Check sheet for the modelled part. Datum: model origin and axes. Units: mm. Face numbers are marked on the shaded views. A direction names the side the tool comes from. Coordinates: 2 decimals unless noted, no trailing zeros. Loops run counter-clockwise (first coordinate to the right, second up) from the corner with the lowest first, then second, coordinate; pieces in that order, holes last.
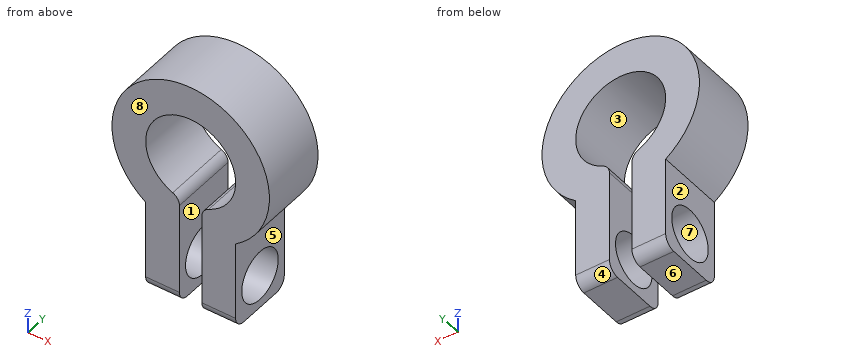
from build123d import *

# Parameters (mm, degrees)
BOSS_EXTRUDE1_DEPTH = 6
SKETCH3_R           = 2.25
CUT_EXTRUDE1_DEPTH  = 10
FILLET1_R           = 1


with BuildPart() as part:
    # Sketch2 → Boss-Extrude1 (new body)
    with BuildSketch(Plane(origin=(0, 0, 0), x_dir=(1, 0, 0), z_dir=(0, 1, 0))):
        with BuildLine():
            Line((-1, 3.872983346), (-1, 13.744562647))
            Line((-1, 13.744562647), (-4, 13.744562647))
            Line((-4, 13.744562647), (-4, 5.744562647))
            ThreePointArc((-4, 5.744562647), (0, -7), (4, 5.744562647))
            Line((4, 5.744562647), (4, 13.744562647))
            Line((4, 13.744562647), (1, 13.744562647))
            Line((1, 13.744562647), (1, 3.872983346))
            ThreePointArc((1, 3.872983346), (0, -4), (-1, 3.872983346))
        make_face()
    extrude(amount=BOSS_EXTRUDE1_DEPTH)

    # Sketch3 → Cut-Extrude1 (cut)
    with BuildSketch(Plane(origin=(4, 0, 0), x_dir=(0, 0, -1), z_dir=(1, 0, 0))):
        with Locations((10.744562647, 3)):
            Circle(SKETCH3_R)
    extrude(amount=-CUT_EXTRUDE1_DEPTH, mode=Mode.SUBTRACT)

    # Fillet1
    fillet1_edges = [part.edges().sort_by_distance(p)[0] for p in [
        (-2.5, 0, -13.744562647),
        (-2.5, 6, -13.744562647),
        (1, 3, -3.872983346),
        (-1, 3, -3.872983346),
        (2.5, 6, -13.744562647),
        (2.5, 0, -13.744562647),
    ]]
    fillet(fillet1_edges, radius=FILLET1_R)


solid = part.part
(1) Draft check along Y on the marked faces 6, 7 and 8. Enter one of: pulls with the +Y half, pulls with the -Y half, needs draft (parallel to the pull), parting line crosses it, or undercut.
(2) Section check D-D, the plane x = -1.25. Enter the section's corners in (y, z), plus the area to 3 significant figures.
(3) Scan lines: line 1 along X through (y, z) = (5.3, -11); line 2 along Z through (x, y) = (-1.75, 1.55); line 3 along X through (y, z) = (2.35, 0). Record each from-to range of solid material in increasing order.
(4) Section check B-B, the plane y = 3. Enter the section's corners in (x, z).
(5) Section check A-A, the plane z = 0. Enter the section's corners in (x, y).
(6) Gauge pin test, flat ends, axial feed: P1, Ø1.5, axis at x = -2, y = 3.5, coming from the +Z side; P2, Ø3, axis at x = -3, y = 3, coming from the +Z side; P3, Ø1.8, axis at y = 2, z = -8.5, coming from the -X side; P4, Ø2.5, axis at y = 3, z = -10.74, coming from the +X side. Record the tip position at first contact, or that the pin passes through.
(7) Set-up check for the marked faces 1, 2, 3, 4 and 5: record each of +Z, -Z, +X, -X, +Y, -Y from which the full face is reachable in a straight line by a thin tool's end or side.
(8) Section check C-C, the plane x = 2.25. Enter the section's corners in (y, z), plus the area to 3 significant figures.
Determined:
1. face 6: needs draft
1. face 7: undercut
1. face 8: pulls with the -Y half
2. outline: (0, -12.74) arc R1 ccw to (1, -13.74) - (5, -13.74) arc R1 ccw to (6, -12.74) - (6, -3.92) - (0, -3.92) - close; (0, 3.8) - (6, 3.8) - (6, 6.89) - (0, 6.89) - close; hole circle Ø4.5 at (3, -10.74)
2. area: 61.1 mm2
3. line 1: x = -4 to -1, 1 to 4
3. line 2: z = -13.74 to -12.47, -9.02 to -3.6, 3.6 to 6.78
3. line 3: x = -7 to -4, 4 to 7
4. outline: (-4, -13.74) - (-1, -13.74) - (-1, -12.99) - (-4, -12.99) - close; (-4, -8.49) - (-1, -8.49) - (-1, -4.58) arc R1 ccw to (-1.6, -3.67) arc R4 cw (long way) to (1.6, -3.67) arc R1 ccw to (1, -4.58) - (1, -8.49) - (4, -8.49) - (4, -5.74) arc R7 ccw (long way) to (-4, -5.74) - close; (1, -13.74) - (4, -13.74) - (4, -12.99) - (1, -12.99) - close
5. outline: (-7, 0) - (-4, 0) - (-4, 6) - (-7, 6) - close; (4, 0) - (7, 0) - (7, 6) - (4, 6) - close
6. P1: stops at z = 6.89
6. P2: stops at z = 6.84
6. P3: stops at x = -4
6. P4: passes through
7. face 1: -Z, +Y, -Y
7. face 2: -Z, -X, +Y, -Y
7. face 3: +Y, -Y
7. face 4: -Z, +X, -X, +Y
7. face 5: -Z, +X, +Y, -Y
8. outline: (0, -12.74) arc R1 ccw to (1, -13.74) - (5, -13.74) arc R1 ccw to (6, -12.74) - (6, -3.31) - (0, -3.31) - close; (0, 3.31) - (6, 3.31) - (6, 6.63) - (0, 6.63) - close; hole circle Ø4.5 at (3, -10.74)
8. area: 66.2 mm2
